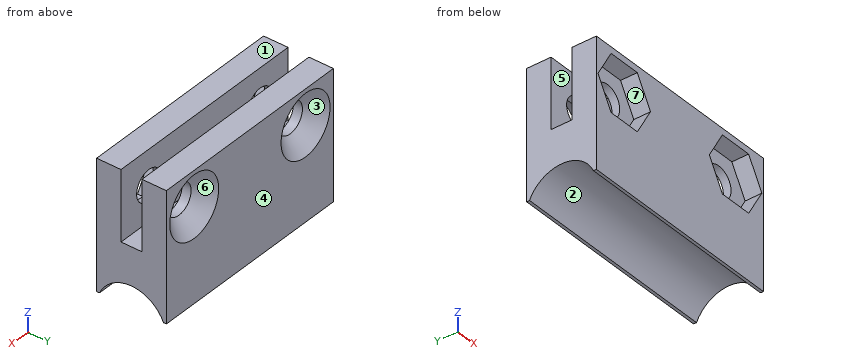
from build123d import *

# Parameters (mm, degrees)
EXTRUDE_1_DEPTH             = 15
SKETCH_2_W                  = 1
SKETCH_2_H                  = 1
CUT_EXTRUDE_1_DEPTH         = 15
HOLE_WIZARD_M21_D           = 2.2
HOLE_WIZARD_M21_CSINK_D     = 4.4
HOLE_WIZARD_M21_CSINK_ANGLE = 90
CUT_EXTRUDE_2_DEPTH         = 1.2


with BuildPart() as part:
    # Эскиз1 → Бобышка-Вытянуть1 (new body)
    with BuildSketch(Plane(origin=(0, 0, 0), x_dir=(0, 0, -1), z_dir=(1, 0, 0))):
        with BuildLine():
            ThreePointArc((10.2, 2.5), (7.7, 0), (10.2, -2.5))
            Line((10.2, -2.5), (0, -2.5))
            Line((0, -2.5), (0, -0.75))
            Line((0, -0.75), (5, -0.75))
            Line((5, -0.75), (5, 0.75))
            Line((5, 0.75), (0, 0.75))
            Line((0, 0.75), (0, 2.5))
            Line((0, 2.5), (10.2, 2.5))
        make_face()
    extrude(amount=EXTRUDE_1_DEPTH)

    # Эскиз2 → Вырез-Вытянуть1 (cut)
    with BuildSketch(Plane(origin=(15, 0, 0), x_dir=(0, 0, -1), z_dir=(1, 0, 0))):
        with Locations((9.7, 2)):
            Rectangle(SKETCH_2_W, SKETCH_2_H)
        with Locations((9.7, -2)):
            Rectangle(SKETCH_2_W, SKETCH_2_H)
    extrude(amount=-CUT_EXTRUDE_1_DEPTH, mode=Mode.SUBTRACT)

    # Зенковка для винта с полупотайной головкой M21 (through all)
    with Locations(Plane(origin=(0, 2.5, 0), x_dir=(1, 0, 0), z_dir=(0, 1, 0))):
        with Locations((12.5, 2.5), (2.5, 2.5)):
            CounterSinkHole(HOLE_WIZARD_M21_D / 2, HOLE_WIZARD_M21_CSINK_D / 2, counter_sink_angle=HOLE_WIZARD_M21_CSINK_ANGLE)

    # Эскиз5 → Вырез-Вытянуть2 (cut)
    with BuildSketch(Plane.XZ.offset(2.5)):
        Polygon((1.321132129, -0.458141777), (0.142264973, -2.500000412), (1.321132843, -4.541858635), (3.678867871, -4.541858223), (4.857735027, -2.499999588), (3.678867157, -0.458141365), align=None)
        Polygon((13.678867157, -4.541858635), (11.321132129, -4.541858223), (10.142264973, -2.499999588), (11.321132843, -0.458141365), (13.678867871, -0.458141777), (14.857735027, -2.500000412), align=None)
    extrude(amount=-CUT_EXTRUDE_2_DEPTH, mode=Mode.SUBTRACT)


solid = part.part
Here's how the part is built. I have some questions about the finished solid (model axes, mm). Face numbers are marked on the shaded views. A direction names the side the tool comes from. Coordinates: 2 decimals unless noted, no trailing zeros. Loops run counter-clockwise (first coordinate to the right, second up) from the corner with the lowest first, then second, coordinate; pieces in that order, holes last.
1. Imagine slicing it at A-A, the plane x = 12.5. Please give me the cut outline in (y, z), and give its area (3 significant figures).
2. I need wall thicknesses on L1, parallel to Y at x = 5.75, z = -3.5; L2, parallel to X at y = 1.9, z = -3.25; L3, parallel to X at y = -1.95, z = -4.5. Which ranges of each line are inside material? Lowest first, please.
3. For the marked faces 5, 6 and 7, which set-ups out of +Z, -Z, +X, -X, +Y, -Y let a thin tool reach every point of the face, with its end or its side?
4. Imagine slicing it at C-C, the plane y = -1.15. Please give me the cut outline in (x, z).
5. For P1, Ø1.8, axis at x = 12.5, z = -2.5, coming from the -Y side; P2, Ø1, axis at x = 13.5, y = 0, coming from the -Z side; P3, Ø1, axis at x = 12.5, y = -1.5, coming from the -Z side, each with a flat end and sliding along its axis, tell me the tip position at first contact or that it passes through.
6. Imagine slicing it at D-D, the plane z = -3.25. Count the separate pieces of the cut face and the enclosed holes in it, and give its area (3 significant figures).
7. Imagine slicing it at B-B, the plane z = -8. Please give me the cut outline in (x, y), and give its area (3 significant figures).
8. If we mould it in two halves opening along Z, with no side actions, what happens to the marked faces 1, 2, 3 and 4? For each: pulls with the +Z half, pulls with the -Z half, needs draft (parallel to the pull), parting line crosses it, or undercut.
Taken from the geometry:
1. outline: (-2.5, -9.2) - (-2.29, -9.2) arc R2.5 cw to (2.29, -9.2) - (2.5, -9.2) - (2.5, -4.7) - (1.4, -3.6) - (0.75, -3.6) - (0.75, -5) - (-0.75, -5) - (-0.75, -3.6) - (-1.3, -3.6) - (-1.3, -4.54) - (-2.5, -4.54) - close; (-2.5, -0.46) - (-1.3, -0.46) - (-1.3, -1.4) - (-0.75, -1.4) - (-0.75, 0) - (-2.5, 0) - close; (0.75, -1.4) - (1.4, -1.4) - (2.5, -0.3) - (2.5, 0) - (0.75, 0) - close
1. area: 22.4 mm2
2. L1: y = -2.5 to -0.75, 0.75 to 2.5
2. L2: x = 0 to 1.09, 3.91 to 11.09, 13.91 to 15
2. L3: x = 0 to 1.3, 3.7 to 11.3, 13.7 to 15
3. face 5: +Z, +X, -X
3. face 6: +Y
3. face 7: -Y
4. outline: (0, -7.98) - (15, -7.98) - (15, 0) - (0, 0) - close; hole circle Ø2.2 at (2.5, -2.5); hole circle Ø2.2 at (12.5, -2.5)
5. P1: passes through
5. P2: stops at z = -7.75
5. P3: stops at z = -8.7
6. separate pieces: 6
6. enclosed holes: 0
6. area: 33.0 mm2
7. outline: (0, -2.5) - (15, -2.5) - (15, -1.19) - (0, -1.19) - close; (0, 1.19) - (15, 1.19) - (15, 2.5) - (0, 2.5) - close
7. area: 39.4 mm2
8. face 1: pulls with the +Z half
8. face 2: pulls with the -Z half
8. face 3: undercut
8. face 4: needs draft
